Part model, mm, in its own coordinate system. Coordinates: 2 decimals unless noted, no trailing zeros. Order: outer loops, then holes, each group sorted by start corner. A loop starts at its lowest first (then second) coordinate and runs counter-clockwise, first axis right, second up. Notation, with made-up numbers: (35.5, -1) - (91.5, -1) arc R26 ccw to (91.5, 13) - close; hole circle Ø2 at (81, -7). An arc over 180 degrees is marked (long way). Use a Markdown table: item, result. Add a question column.
1) Saw through at A-A on y = -3. List the corners of the cut face in (x, z).
2) Drop a flat-ended pin along its axis: P1, Ø10, axis at y = 4, z = 15.5, coming from the +X side. Give the stop position or say it passes through.
3) Saw through at C-C on z = 12.25. List the corners of the cut face in (x, y), then the cut area to 3 significant figures.
4) Saw through at B-B on z = 15.5. List the corners of the cut face in (x, y).
5) Wall check: L1, parallel to X at y = -24.5, z = 15; L2, parallel to Z at x = -22.5, y = 18; L3, parallel to X at y = 23, z = 9.25. Give the ranges that are in metal, low to high. Write a range as [from, to].
```python
from build123d import *

# Parameters (mm, degrees)
SKETCH1_W           = 58.5
SKETCH1_H           = 62
BOSS_EXTRUDE1_DEPTH = 18
FILLET1_R           = 10


with BuildPart() as part:
    # Sketch1 → Boss-Extrude1 (new body)
    with BuildSketch(Plane.XY):
        Rectangle(SKETCH1_W, SKETCH1_H)
    extrude(amount=BOSS_EXTRUDE1_DEPTH)

    # Fillet1
    fillet1_edges = [part.edges().sort_by_distance(p)[0] for p in [
        (-29.25, 0, 18),
        (29.25, 0, 18),
    ]]
    fillet(fillet1_edges, radius=FILLET1_R)


solid = part.part
```
Results are:
| question | item | result |
|---|---|---|
| 1 | outline | (-29.25, 0) - (29.25, 0) - (29.25, 8) arc R10 ccw to (19.25, 18) - (-19.25, 18) arc R10 ccw to (-29.25, 8) - close |
| 2 | P1 | x = 28.93 |
| 3 | outline | (-28.3, -31) - (28.3, -31) - (28.3, 31) - (-28.3, 31) - close |
| 3 | area | 3,510 mm2 |
| 4 | outline | (-25.86, -31) - (25.86, -31) - (25.86, 31) - (-25.86, 31) - close |
| 5 | L1 | [-26.39, 26.39] |
| 5 | L2 | [0, 17.46] |
| 5 | L3 | [-29.17, 29.17] |
